CAD build for the part. Positions are in the model's coordinates, mm. Round coordinates to 2 decimals unless told otherwise and drop trailing zeros. Loops run counter-clockwise (first coordinate to the right, second up) from the corner with the lowest first, then second, coordinate; pieces in that order, holes last. Notation, with made-up numbers: (71, 12.25) -> (77, 12.25) arc R14 cw to (77, 39.25) -> close; hole circle Ø9 at (86.5, 49.5). An arc over 180 degrees is marked (long way). Answer as CSV lines item,"result".
```python
from build123d import *

# Parameters (mm, degrees)
BOSS_EXTRUDE1_DEPTH = 3
SKETCH3_W           = 8.2
SKETCH3_H           = 3.2
SKETCH3_W_2         = 3.2
SKETCH3_H_2         = 8.2
CUT_EXTRUDE3_DEPTH  = 4


with BuildPart() as part:
    # Sketch1 → Boss-Extrude1 (new body)
    with BuildSketch(Plane.XY):
        Polygon((0, 52.125), (11.2, 52.125), (11.2, 43.925), (16.5, 43.925), (16.5, 40.925), (63.5, 40.925), (63.5, 43.925), (68.8, 43.925), (68.8, 52.125), (80, 52.125), (80, 3.175), (64, 3.175), (64, 15.625), (16, 15.625), (16, 3.175), (0, 3.175), align=None)
    extrude(amount=-BOSS_EXTRUDE1_DEPTH)

    # Sketch3 → Cut-Extrude3 (cut, through all)
    with BuildSketch(Plane.XY):
        with Locations((40, 17.125)):
            Rectangle(SKETCH3_W, SKETCH3_H)
        with Locations((56, 17.125)):
            Rectangle(SKETCH3_W, SKETCH3_H)
        with Locations((24, 17.125)):
            Rectangle(SKETCH3_W, SKETCH3_H)
        with Locations((78.5, 12.925)):
            Rectangle(SKETCH3_W_2, SKETCH3_H_2)
        Polygon((3.1, 40.825), (3.1, 49.025), (8.1, 49.025), (8.1, 40.825), (71.9, 40.825), (71.9, 49.025), (76.9, 49.025), (76.9, 40.825), (80.1, 40.825), (80.1, 52.225), (68.7, 52.225), (68.7, 44.025), (11.3, 44.025), (11.3, 52.225), (-0.1, 52.225), (-0.1, 40.825), align=None)
        with Locations((28.5, 28.925)):
            Rectangle(SKETCH3_W_2, SKETCH3_H_2)
        with Locations((8, 4.675)):
            Rectangle(SKETCH3_W, SKETCH3_H)
        with Locations((1.5, 12.925)):
            Rectangle(SKETCH3_W_2, SKETCH3_H_2)
        with Locations((1.5, 28.925)):
            Rectangle(SKETCH3_W_2, SKETCH3_H_2)
        with Locations((78.5, 28.925)):
            Rectangle(SKETCH3_W_2, SKETCH3_H_2)
        with Locations((72, 4.675)):
            Rectangle(SKETCH3_W, SKETCH3_H)
    extrude(amount=-CUT_EXTRUDE3_DEPTH, mode=Mode.SUBTRACT)


solid = part.part
```
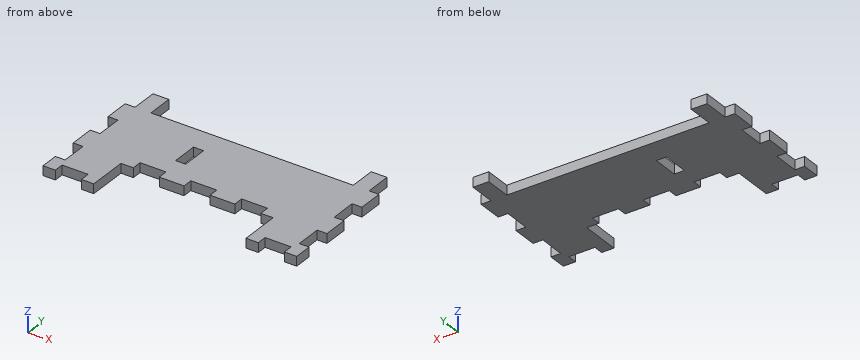
Q1. Slice it at B-B, the plane x = 70.5. Give the cut face in (y, z) (3 decimals), and give its area (3 significant figures).
Results:
outline,"(6.275, -3) -> (40.825, -3) -> (40.825, 0) -> (6.275, 0) -> close"
area,"104 mm2"
Q2. Slice it at A-A, the plane x = 39.5. Give the cut face in (y, z) (3 decimals), and give its area (3 significant figures).
Results:
outline,"(18.725, -3) -> (40.825, -3) -> (40.825, 0) -> (18.725, 0) -> close"
area,"66.3 mm2"
Q3. Drop flat-ended pins along their axis: pin 1 Ø0.9 at (x, z) = (24, -1) entering from -Y (3 decimals); pin 2 Ø1.5 at (y, z) = (30, -1.5) entering from -X; pin 3 Ø0.9 at (x, z) = (6, -1.5) entering from -Y (3 decimals). Give the stop position or say it passes through.
Results:
pin 1,"y = 18.725"
pin 2,"x = 3.1"
pin 3,"y = 6.275"
Q4. Probe L1, parallel to X at y = 32, z = -1.3; L2, parallel to X at y = 13.5, z = -1.4; L3, parallel to Y at x = 36.5, z = -1.8 (3 decimals). List the from-to ranges inside material, lowest first. Write a range as [from, to].
Results:
L1,"[3.1, 26.9], [30.1, 76.9]"
L2,"[3.1, 16], [64, 76.9]"
L3,"[18.725, 40.825]"
